```python
from build123d import *

# Parameters (mm, degrees)
SKETCH2_R           = 4.7625
BOSS_EXTRUDE1_DEPTH = 3.175
SKETCH5_R           = 1.27
CUT_EXTRUDE1_DEPTH  = 7.35
CUT_EXTRUDE2_START  = 1.905
CUT_EXTRUDE2_DEPTH  = 3.8575
CIRPATTERN2_COUNT   = 12


with BuildPart() as part:
    # Sketch2 → Boss-Extrude1 (new body, symmetric)
    with BuildSketch(Plane.XY):
        Circle(SKETCH2_R)
    extrude(amount=BOSS_EXTRUDE1_DEPTH, both=True)

    # Sketch5 → Cut-Extrude1 (cut, through all)
    with BuildSketch(Plane(origin=(0, 0, -3.175), x_dir=(-1, 0, 0), z_dir=(0, 0, -1))):
        Circle(SKETCH5_R)
    extrude(amount=-CUT_EXTRUDE1_DEPTH, mode=Mode.SUBTRACT)

    # Sketch4_2 → Cut-Extrude2 (cut, through all)
    with BuildSketch(Plane(origin=(0, 0, 0), x_dir=(1, 0, 0), z_dir=(0, 1, 0)).offset(CUT_EXTRUDE2_START)):
        with BuildLine():
            Line((-0.108840568, -3.556), (-3.918840568, 1.524))
            Line((-3.918840568, 1.524), (-3.410840568, 1.905))
            Line((-3.410840568, 1.905), (0.399159432, -3.175))
            ThreePointArc((0.399159432, -3.175), (0.335659432, -3.6195), (-0.108840568, -3.556))
        make_face()
    cut_extrude2 = extrude(amount=CUT_EXTRUDE2_DEPTH, mode=Mode.SUBTRACT)

    # CirPattern2: Cut-Extrude2 ×12 about axis
    cirpattern2_axis = Axis((0, 0, 0), (0, 0, 1))
    for i in range(1, CIRPATTERN2_COUNT):
        add(cut_extrude2.rotate(cirpattern2_axis, i * 360 / CIRPATTERN2_COUNT), mode=Mode.SUBTRACT)


solid = part.part
```
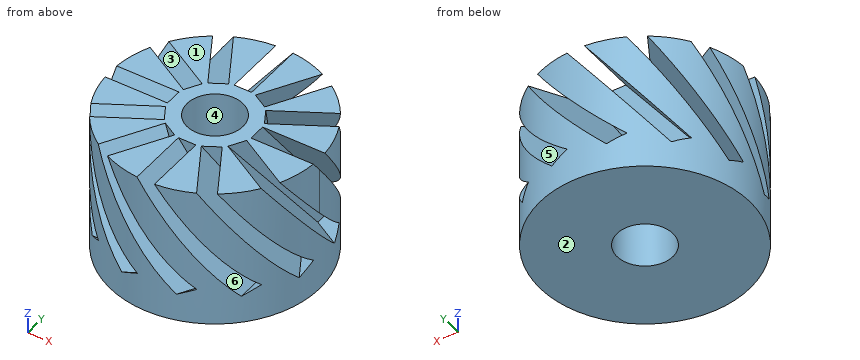
Work out the finished part from the listing and answer in its coordinate system (mm). Face numbers are marked on the shaded views. A direction names the side the tool comes from. Coordinates: 2 decimals unless noted, no trailing zeros. Use a Markdown table: item, result.
Item 1: For the marked faces 5 and 6, determine the directions among +Z, -Z, +X, -X, +Y, -Y from which every point of the face is accessible in a straight line to the end or side of a thin tool.
Evaluation:
| item | result |
|---|---|
| face 5 | none |
| face 6 | -Y |
Item 2: Given pin 1 Ø1 at (y, z) = (-2.5, 2.5) entering from +X; pin 2 Ø2 at (y, z) = (-1.5, 1.5) entering from -X; pin 3 Ø3.5 at (x, z) = (3, 1) entering from -Y, each flat-ended and moving along its own axis, determine where each tip first touches the part or whether it passes through.
Evaluation:
| item | result |
|---|---|
| pin 1 | stops at x = 4.28 |
| pin 2 | stops at x = -4.74 |
| pin 3 | stops at y = -4.6 |
Item 3: Consider probe 1 along Y at (x, z) = (0, -1.5); probe 2 along Z at (x, y) = (3.5, 2) (3 decimals); probe 3 along Y at (x, z) = (0, 0.75). Determine where each line is inside the solid, lowest interval first. Write a range as from..to.
Evaluation:
| item | result |
|---|---|
| probe 1 | y = -4.76..-4.5, -3.81..-1.27, 1.27..3.81, 4.5..4.76 |
| probe 2 | z = -3.175..-1.852, -0.942..-0.024, 1.034..2.667 |
| probe 3 | y = -4.76..-4.43, -2.84..-1.27, 1.27..2.84, 4.43..4.76 |
Item 4: The mould has two halves that part along Z. Classify the marked faces 1, 2, 3 and 4: +Z half, -Z half, draft (parallel to the pull), parting line (faces both ways), or undercut.
Evaluation:
| item | result |
|---|---|
| face 1 | +Z half |
| face 2 | -Z half |
| face 3 | undercut |
| face 4 | draft |
